Work out the finished part from the listing and answer in its coordinate system (mm). A direction names the side the tool comes from. Coordinates: 2 decimals unless noted, no trailing zeros. Order: outer loops, then holes, each group sorted by start corner. A loop starts at its lowest first (then second) coordinate and runs counter-clockwise, first axis right, second up. Notation, with made-up numbers: M -11.75,-6.5 L 35.25,-6.5 A20 cw 35.25,3.5 Z; hole C -30,-27.75 d1. An arc over 180 degrees is marked long. Use a Markdown table: item, result.
from build123d import *

# Parameters (mm, degrees)
F1_DEPTH = 76.2


with BuildPart() as f1:
    # F0 (on Front) → F1 (new body)
    with BuildSketch(Plane.XZ):
        with BuildLine():
            Line((-75.81626, -39.602265), (-75.511565, -72.197098))
            ThreePointArc((-75.511565, -72.197098), (-45.783731, -66.25503), (-31.337889, -39.602265))
            Line((-31.337889, -39.602265), (-45.608908, -39.602265))
            Line((-45.608908, -39.602265), (-63.353062, -39.602265))
            Line((-63.353062, -39.602265), (-75.81626, -39.602265))
        make_face()
        Polygon((-63.353062, -39.602265), (-45.608908, -39.602265), (-45.608908, -18.955742), (-63.353062, -18.955742), (-73.227495, -18.955742), (-73.227495, -27.083755), (-63.353062, -27.083755), align=None)
    extrude(amount=F1_DEPTH)


solid = f1.part
(1) Straight lines are drawn through the part: L1, parallel to Z at x = -66.5, y = -29; L2, parallel to X at y = -60.5, z = -26.5; L3, parallel to X at y = -53.5, z = -37.5. For each, find the intervals that lie inside material, in ascending order.
Conclusion:
| item | result |
|---|---|
| L1 | -73.23 to -39.6, -27.08 to -18.96 |
| L2 | -73.23 to -45.61 |
| L3 | -63.35 to -45.61 |
(2) Given P1, Ø6.5, axis at y = -48, z = -32, coming from the -X side; P2, Ø6, axis at x = -61.5, y = -32, coming from the -Z side; P3, Ø1.5, axis at y = -50, z = -60, coming from the +X side, each flat-ended and moving along its own axis, determine where each tip first touches the part or whether it passes through.
Conclusion:
| item | result |
|---|---|
| P1 | x = -63.35 |
| P2 | z = -73.14 |
| P3 | x = -38.65 |
(3) Determine the mould class of faces 1 (the cylindrical face through (-46.138, -37.567, -66.513)), 2 (the flat face through (-59, -38, -18.956)), 3 (the flat face through (-68, -38, -27.084)) for opening direction Z: pulls with the +Z half, pulls with the -Z half, needs draft (parallel to the pull), parting line crosses it, or undercut.
Conclusion:
| item | result |
|---|---|
| face 1 | pulls with the -Z half |
| face 2 | pulls with the +Z half |
| face 3 | undercut |
(4) A cutting plane is placed at A-A (y = -15.5). Determine the outline of the cut face in (x, z).
Conclusion:
| item | result |
|---|---|
| outline | M -75.82,-39.6 L -75.51,-72.2 A35.71 ccw -31.34,-39.6 L -45.61,-39.6 L -45.61,-18.96 L -73.23,-18.96 L -73.23,-27.08 L -63.35,-27.08 L -63.35,-39.6 Z |
(5) A cutting plane is placed at B-B (x = -40). Determine the outline of the cut face in (y, z), then the cut area to 3 significant figures.
Conclusion:
| item | result |
|---|---|
| outline | M -76.2,-60.91 L 0,-60.91 L 0,-39.6 L -76.2,-39.6 Z |
| area | 1,620 mm2 |
(6) A cutting plane is placed at C-C (z = -59). Determine the outline of the cut face in (x, y).
Conclusion:
| item | result |
|---|---|
| outline | M -75.63,-76.2 L -38.46,-76.2 L -38.46,0 L -75.63,0 Z |
(7) Which of the six approach directions +Z, -Z, +X, -X, +Y, -Y give full straight-line access (tool end or side, diameter ignored) to faces 4 (the flat face through (-45.609, -38, -29)), 5 (the flat face through (-73.227, -38, -23)), 6 (the flat face through (-59, -76.2, -46)), 7 (the flat face through (-69, -38, -39.602))?
Conclusion:
| item | result |
|---|---|
| face 4 | +Z, +X, +Y, -Y |
| face 5 | +Z, -X, +Y, -Y |
| face 6 | +Z, -Z, +X, -X, -Y |
| face 7 | -X, +Y, -Y |
